from build123d import *

# Parameters (mm, degrees)
SKETCH_1_W      = 85.8
SKETCH_1_H      = 60
SKETCH_1_W_2    = 58.5
SKETCH_1_H_2    = 39.4
EXTRUDE_1_DEPTH = 0.6
SKETCH_2_W      = 2
SKETCH_2_H      = 58
SKETCH_2_W_2    = 81.8
SKETCH_2_H_2    = 2
EXTRUDE_2_DEPTH = 2
FILLET_1_R      = 1


with BuildPart() as part:
    # 草图1 → 凸台-拉伸1 (new body)
    with BuildSketch(Plane.XY):
        Rectangle(SKETCH_1_W, SKETCH_1_H)
        with Locations((9.15, 0.2)):
            Rectangle(SKETCH_1_W_2, SKETCH_1_H_2, mode=Mode.SUBTRACT)
    extrude(amount=EXTRUDE_1_DEPTH)

    # 草图2 → 凸台-拉伸2 (add)
    with BuildSketch(Plane(origin=(0, 0, 0), x_dir=(-1, 0, 0), z_dir=(0, 0, -1))):
        with Locations((-41.9, 1)):
            Rectangle(SKETCH_2_W, SKETCH_2_H)
        with Locations((0, -29)):
            Rectangle(SKETCH_2_W_2, SKETCH_2_H_2)
        with Locations((-41.9, -29)):
            Rectangle(SKETCH_2_W, SKETCH_2_H_2)
        with Locations((41.9, 1)):
            Rectangle(SKETCH_2_W, SKETCH_2_H)
        with Locations((41.9, -29)):
            Rectangle(SKETCH_2_W, SKETCH_2_H_2)
    extrude(amount=EXTRUDE_2_DEPTH)

    # 圆角1
    fillet_1_edges = [part.edges().sort_by_distance(p)[0] for p in [
        (42.9, -30, -0.7),
        (-42.9, -30, -0.7),
    ]]
    fillet(fillet_1_edges, radius=FILLET_1_R)


solid = part.part
Verification items for the finished model (mm, model axes). A direction names the side the tool comes from. Give positions to 0.01 mm unless a question says otherwise; leave off trailing zeros. Loops run counter-clockwise (first coordinate to the right, second up) from the corner with the lowest first, then second, coordinate; pieces in that order, holes last.
1) Set-up check for faces 5 (the flat face through (0.2, 30, 0.2)), 6 (the flat face through (40.9, 1, -1)): record each of +Z, -Z, +X, -X, +Y, -Y from which the full face is reachable in a straight line by a thin tool's end or side.
2) Draft check along X on faces 1 (the flat face through (-40.9, 1, -1)), 2 (the flat face through (-10, 21, 0)), 3 (the flat face through (0, -29, -2)), 4 (the flat face through (42.9, 1, -1)). Enter one of: pulls with the +X half, pulls with the -X half, needs draft (parallel to the pull), parting line crosses it, or undercut.
3) Depth check by flat-ended pin: pin 1 Ø1 at (x, y) = (-18, 12.5) entering from +Z. Enter the tip coordinate at first touch or a pass-through.
4) Sectioned sample at B-B, the plane x = 32. Enter the section's corners in (y, z), then the cut area to 3 significant figures.
5) Sectioned sample at C-C, the plane z = -1.2. Enter the section's corners in (x, y).
6) Thickness scan on line 1 along X through (y, z) = (-2, -0.45); line 2 along Y through (x, z) = (-9, 0.5); line 3 along X through (y, z) = (18, 0.25). Record the ranges inside material, lowest first.
7) Sectioned sample at D-D, the plane x = -23. Enter the section's corners in (y, z).
8) Sectioned sample at A-A, the plane y = 18.5. Enter the section's corners in (x, z), then the cut area to 3 significant figures.
Answers:
1. face 5: +Z, -Z, +X, -X, +Y
1. face 6: -Z, +Y
2. face 1: undercut
2. face 2: undercut
2. face 3: needs draft
2. face 4: pulls with the +X half
3. pin 1: passes through
4. outline: (-30, -2) - (-28, -2) - (-28, 0) - (-19.5, 0) - (-19.5, 0.6) - (-30, 0.6) - close; (19.9, 0) - (30, 0) - (30, 0.6) - (19.9, 0.6) - close
4. area: 16.4 mm2
5. outline: (-42.9, -29) arc R1 ccw to (-41.9, -30) - (41.9, -30) arc R1 ccw to (42.9, -29) - (42.9, 30) - (40.9, 30) - (40.9, -28) - (-40.9, -28) - (-40.9, 30) - (-42.9, 30) - close
6. line 1: x = -42.9 to -40.9, 40.9 to 42.9
6. line 2: y = -30 to -19.5, 19.9 to 30
6. line 3: x = -42.9 to -20.1, 38.4 to 42.9
7. outline: (-30, -2) - (-28, -2) - (-28, 0) - (30, 0) - (30, 0.6) - (-30, 0.6) - close
8. outline: (-42.9, -2) - (-40.9, -2) - (-40.9, 0) - (-20.1, 0) - (-20.1, 0.6) - (-42.9, 0.6) - close; (38.4, 0) - (40.9, 0) - (40.9, -2) - (42.9, -2) - (42.9, 0.6) - (38.4, 0.6) - close
8. area: 24.4 mm2
